Read the model definition and answer for the solid it produces. Units are mm, in the model's axes. Face numbers are marked on the shaded views. A direction names the side the tool comes from. Give positions to 0.01 mm unless a question says otherwise; leave off trailing zeros. Write each loop counter-clockwise with the first axis right and the second up, starting at its lowest first coordinate (ties: lowest second). Pieces come first, ordered by that corner, then holes. Notation, with made-up numbers: (82.5, 52.25) - (133.5, 52.25) arc R25 ccw to (133.5, 74.25) - close; hole circle Ø7 at (39.5, 56.5). An arc over 180 degrees is marked (long way). Answer as a JSON object with one key per item and string values. Group by question number.
```python
from build123d import *

# Parameters (mm, degrees)
F0_W     = 7
F0_H     = 10
F0_R     = 1.6
F1_DEPTH = 3
F0_H_2   = 5
F2_DEPTH = 12
F4_DEPTH = 25
F5_DEPTH = 7
F6_R     = 1.5
F7_DEPTH = 10


with BuildPart() as f1:
    # F0 (on Top) → F1 (new body)
    with BuildSketch(Plane.XY):
        with Locations((-3.5, -5)):
            Rectangle(F0_W, F0_H)
        with Locations((-3.5, -3)):
            Circle(F0_R, mode=Mode.SUBTRACT)
    extrude(amount=F1_DEPTH)

    # F0 (on Top) → F2 (join)
    with BuildSketch(Plane.XY):
        with Locations((-3.5, -12.5)):
            Rectangle(F0_W, F0_H_2)
    extrude(amount=F2_DEPTH)

    # F3 (on face) → F4 (cut)
    with BuildSketch(Plane(origin=(-7, 0, 0), x_dir=(0, -1, 0), z_dir=(-1, 0, 0))):
        Polygon((10.1929933606, 11.5368159345), (15, 0), (15, 12), (10, 12), align=None)
        Polygon((10, 11.4564020342), (10.1929933606, 11.5368159345), (10, 12), align=None)
    extrude(amount=-F4_DEPTH, mode=Mode.SUBTRACT)

    # F3 (on face) → F5 (join)
    with BuildSketch(Plane(origin=(-7, 0, 0), x_dir=(0, -1, 0), z_dir=(-1, 0, 0))):
        Polygon((10, 3), (10, 11.4564020342), (6.9977270885, 10.2054549877), align=None)
    extrude(amount=-F5_DEPTH)

    # F6 (on face) → F7 (cut)
    with BuildSketch(Plane(origin=(0, -12.7810650888, 5.325443787), x_dir=(1, 0, 0), z_dir=(0, -0.9230769231, 0.3846153846))):
        with Locations((-3.5, 3.2289864931)):
            Circle(F6_R)
    extrude(amount=-F7_DEPTH, mode=Mode.SUBTRACT)


solid = f1.part
```
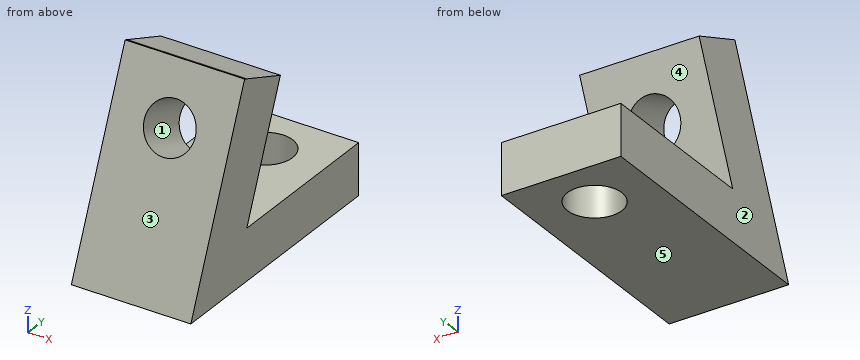
1) Find the intervals of material crossed by line 1 (Z direction, x = -4, y = -6); line 2 (Y direction, x = -3.5, z = 2.45); line 3 (X direction, y = -8.75, z = 8.5), in increasing order. Write a range as [from, to].
2) Find section B-B, the plane x = -2.75. Write down the section's boundary in (y, z).
3) Find section A-A, the plane y = -3. Write down the section's boundary in (x, z), and give its area (3 significant figures).
4) For a pull along X with two mould halves and no side action, classify the marked faces 1, 2 and 3 as released by +X, released by -X, zero draft, split by the parting line, or undercut.
5) Flat-ended cylindrical pins translate along their axes: pin 1 Ø1.5 at (x, z) = (-5, 9.5) entering from +Y; pin 2 Ø3 at (x, z) = (-5.5, 8.5) entering from -Y; pin 3 Ø3 at (x, y) = (-3.5, -3) entering from +Z. Find the tip coordinate at first contact, or state that the pin passes through.
6) Find section D-D, the plane z = 2. Write down the section's boundary in (x, y), and give its area (3 significant figures).
7) Find section C-C, the plane x = -6. Write down the section's boundary in (y, z).
8) Which of the six approach directions +Z, -Z, +X, -X, +Y, -Y give full straight-line access (tool end or side, diameter ignored) to the marked faces 4 and 5?
Values follow:
{
 "1": {"line 1": "z = [0, 3]", "line 2": "y = [-13.98, -4.6], [-1.4, 0]", "line 3": "x = [-7, -4.33], [-2.67, 0]"},
 "2": {"outline": "(-15, 0) - (-4.41, 0) - (-4.41, 3) - (-10, 3) - (-8.84, 5.78) - (-12.04, 7.11) - close; (-11.04, 9.51) - (-7.84, 8.17) - (-7, 10.21) - (-10.19, 11.54) - close; (-1.59, 0) - (0, 0) - (0, 3) - (-1.59, 3) - close"},
 "3": {"outline": "(-7, 0) - (-5.1, 0) - (-5.1, 3) - (-7, 3) - close; (-1.9, 0) - (0, 0) - (0, 3) - (-1.9, 3) - close", "area": "11.4 mm2"},
 "4": {"face 1": "undercut", "face 2": "released by -X", "face 3": "zero draft"},
 "5": {"pin 1": "stops at y = -7", "pin 2": "stops at y = -12.08", "pin 3": "passes through"},
 "6": {"outline": "(-7, -14.17) - (0, -14.17) - (0, 0) - (-7, 0) - close; hole circle Ø3.2 at (-3.5, -3)", "area": "91.1 mm2"},
 "7": {"outline": "(-15, 0) - (0, 0) - (0, 3) - (-10, 3) - (-7, 10.21) - (-10.19, 11.54) - close"},
 "8": {"face 4": "+X, -X, +Y", "face 5": "-Z, +X, -X, +Y, -Y"}
}
